Check sheet for the drawn part. Datum: minimum x, y, z corner. Units: mm. Give positions to 0.01 mm unless a question says otherwise; leave off trailing zeros. Order: outer loops, then holes, each group sorted by start corner. A loop starts at its lowest first (then second) coordinate and runs counter-clockwise, first axis right, second up.
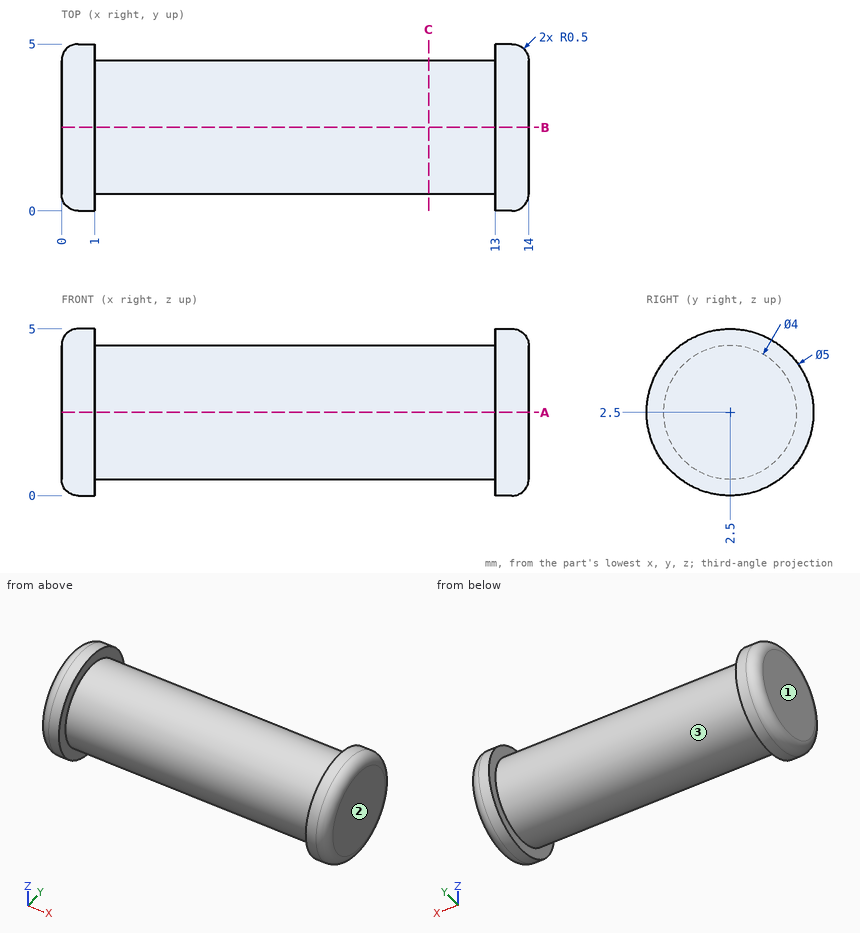
Item 1: Draft check along X on the marked faces 1, 2 and 3. Enter one of: released by +X, released by -X, zero draft, split by the parting line, or undercut.
Reported:
face 1: released by -X
face 2: released by +X
face 3: undercut
Item 2: Scan lines: L1, parallel to X at y = 0.55, z = 3.35; L2, parallel to X at y = 1.1, z = 4.4; L3, parallel to Y at x = 6.5, z = 0.7. Record each from-to range of solid material in increasing order.
Reported:
L1: x = 0.02 to 1, 13 to 13.98
L2: x = 0.15 to 1, 13 to 13.85
L3: y = 1.63 to 3.37
Item 3: Gauge pin test, flat ends, axial feed: pin 1 (1 mm diameter, centred on x = 5, z = 1.5, fed in from +Y); pin 2 (1 mm diameter, centred on x = 9.5, z = 4.5, fed in from +Y). Record the tip position at first contact, or that the pin passes through.
Reported:
pin 1: stops at y = 4.44
pin 2: stops at y = 3.82
Item 4: Sectioned sample at C-C (x = 11). Enter the section's corners in (y, z).
Reported:
outline: circle Ø4 at (2.5, 2.5)
Item 5: Sectioned sample at A-A (z = 2.5). Enter the section's corners in (x, y), and give its area (3 significant figures).
Reported:
outline: (0, 0.5) arc R0.5 ccw to (0.5, 0) - (1, 0) - (1, 0.5) - (13, 0.5) - (13, 0) - (13.5, 0) arc R0.5 ccw to (14, 0.5) - (14, 4.5) arc R0.5 ccw to (13.5, 5) - (13, 5) - (13, 4.5) - (1, 4.5) - (1, 5) - (0.5, 5) arc R0.5 ccw to (0, 4.5) - close
area: 57.8 mm2
